Here's how the part is built. I have some questions about the finished solid (model axes, mm). Face numbers are marked on the shaded views. A direction names the side the tool comes from. Round coordinates to 2 decimals unless told otherwise and drop trailing zeros. Loops run counter-clockwise (first coordinate to the right, second up) from the corner with the lowest first, then second, coordinate; pieces in that order, holes last. Notation, with made-up numbers: M -13.75,80.25 L 14.25,80.25 A33 ccw 14.25,111.25 Z; hole C 82.5,55 d9. An arc over 180 degrees is marked long. Write each question's results on one line, items separated by ' | '. Start each with the question number.
```python
from build123d import *

# Parameters (mm, degrees)
SKETCH3_R           = 1.5
SKETCH3_R_2         = 2.8
BOSS_EXTRUDE1_DEPTH = 4
SKETCH3_3_R         = 4
SKETCH3_3_R_2       = 2.8
BOSS_EXTRUDE2_DEPTH = 10


with BuildPart() as part:
    # Sketch3 → Boss-Extrude1 (new body)
    with BuildSketch(Plane.XY):
        with BuildLine():
            ThreePointArc((-6, -3), (0, -9), (6, -3))
            Line((6, -3), (6, 3))
            ThreePointArc((6, 3), (0, 9), (-6, 3))
            Line((-6, 3), (-6, -3))
        make_face()
        with Locations((0, -6)):
            Circle(SKETCH3_R, mode=Mode.SUBTRACT)
        with Locations((0, 6)):
            Circle(SKETCH3_R, mode=Mode.SUBTRACT)
        Circle(SKETCH3_R_2, mode=Mode.SUBTRACT)
    extrude(amount=BOSS_EXTRUDE1_DEPTH)

    # Sketch3<3> → Boss-Extrude2 (add)
    with BuildSketch(Plane.XY):
        Circle(SKETCH3_3_R)
        Circle(SKETCH3_3_R_2, mode=Mode.SUBTRACT)
    extrude(amount=BOSS_EXTRUDE2_DEPTH)


solid = part.part
```
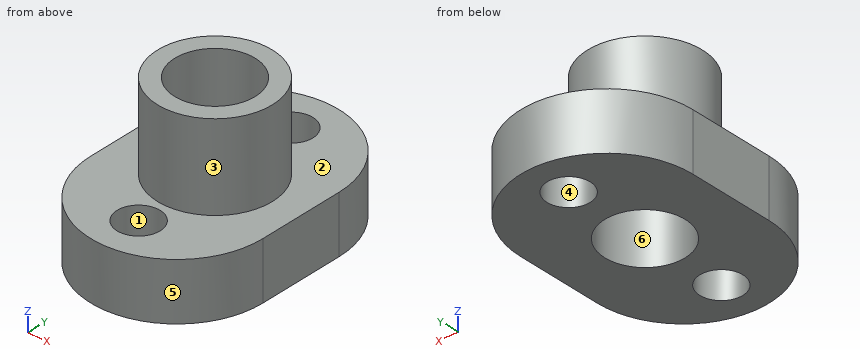
1. I want a section at C-C on x = 0. List the corners of the cut face in (y, z) for me, plus the area to 3 significant figures.
2. If we mould it in two halves opening along Y, with no side actions, what happens to the marked faces 3, 4, 5 and 6? For each: released by +Y, released by -Y, zero draft, split by the parting line, or undercut.
3. I want a section at A-A on y = 0. List the corners of the cut face in (x, z) for me, plus the area to 3 significant figures.
4. I need wall thicknesses on line 1 along Y through (x, z) = (0, 1.35); line 2 along Y through (x, z) = (0, 6.5); line 3 along Z through (x, y) = (1.75, -5.75). Which ranges of each line are inside material? Lowest first, please.
5. Which directions (+Z, -Z, +X, -X, +Y, -Y) give clear straight access to the entire face, cutting with the end or side of a thin tool? Please do the marked faces 1 and 2.
6. I want a section at D-D on y = -3.5. List the corners of the cut face in (x, z) for me, plus the area to 3 significant figures.
7. For pin 1 (1.5 mm diameter, centred on y = -3.5, z = 8.5, fed in from +X); pin 2 (2 mm diameter, centred on x = -3.5, z = 6.5, fed in from -Y); pin 3 (4 mm diameter, centred on x = 4.5, z = 8.5, fed in from +Y); pin 4 (2.5 mm diameter, centred on x = 0, y = 6, fed in from +Z), each with a flat end and sliding along its axis, tell me the tip position at first contact or that it passes through.
8. I want a section at B-B on z = 3.5. List the corners of the cut face in (x, y) for me, plus the area to 3 significant figures.
Outcome:
1) outline: M -9,0 L -7.5,0 L -7.5,4 L -9,4 Z; M -4.5,0 L -2.8,0 L -2.8,10 L -4,10 L -4,4 L -4.5,4 Z; M 2.8,0 L 4.5,0 L 4.5,4 L 4,4 L 4,10 L 2.8,10 Z; M 7.5,0 L 9,0 L 9,4 L 7.5,4 Z | area: 40.0 mm2
2) face 3: split by the parting line | face 4: undercut | face 5: released by -Y | face 6: undercut
3) outline: M -6,0 L -2.8,0 L -2.8,10 L -4,10 L -4,4 L -6,4 Z; M 2.8,0 L 6,0 L 6,4 L 4,4 L 4,10 L 2.8,10 Z | area: 40.0 mm2
4) line 1: -9 to -7.5, -4.5 to -2.8, 2.8 to 4.5, 7.5 to 9 | line 2: -4 to -2.8, 2.8 to 4 | line 3: 0 to 4
5) face 1: +Z, -Z | face 2: +Z
6) outline: M -5.98,0 L 5.98,0 L 5.98,4 L 1.94,4 L 1.94,10 L -1.94,10 L -1.94,4 L -5.98,4 Z | area: 71.1 mm2
7) pin 1: x = 2.9 | pin 2: y = -3.12 | pin 3: y = 3.12 | pin 4: through
8) outline: M -6,-3 A6 ccw 6,-3 L 6,3 A6 ccw -6,3 Z; hole C 0,0 d5.6; hole C 0,-6 d3; hole C 0,6 d3 | area: 146 mm2
